Read the model definition and answer for the solid it produces. Units are mm, in the model's axes. Coordinates: 2 decimals unless noted, no trailing zeros. Answer as a JSON object with one key per item and string values. Group by question number.
1) Consider L1, parallel to Z at x = 114.3, y = -0.5; L2, parallel to Z at x = 193, y = 8. Determine where each line is inside the solid, lowest interval first.
2) Given pin 1 (9.5 mm diameter, centred on x = -38.1, z = 1047.75, fed in from -Y); pin 2 (11 mm diameter, centred on x = 38.1, z = 1047.75, fed in from -Y); pin 3 (13.5 mm diameter, centred on x = 38.1, z = 19.05, fed in from -Y), each flat-ended and moving along its own axis, determine where each tip first touches the part or whether it passes through.
3) Determine the mould class of faces 1 (the flat face through (-3, 0, 1066.8)), 2 (the flat face through (241.3, 0, 526)), 3 (the flat face through (-241.3, 0, 526)) for opening direction X: released by +X, released by -X, zero draft, split by the parting line, or undercut.
from build123d import *

# Parameters (mm, degrees)
SKETCH2_W                                         = 482.6
SKETCH2_H                                         = 38.1
BOSS_EXTRUDE1_DEPTH                               = 1066.8
CSK_FOR_5_16_FLAT_HEAD_MACHINE_SCREW1_D           = 8.4328
CSK_FOR_5_16_FLAT_HEAD_MACHINE_SCREW1_CSINK_D     = 16.129
CSK_FOR_5_16_FLAT_HEAD_MACHINE_SCREW1_CSINK_ANGLE = 82


with BuildPart() as part:
    # Sketch2 → Boss-Extrude1 (new body)
    with BuildSketch(Plane.XY):
        Rectangle(SKETCH2_W, SKETCH2_H)
    extrude(amount=BOSS_EXTRUDE1_DEPTH)

    # CSK for 5/16 Flat Head Machine Screw1 (through all)
    with Locations(Plane(origin=(0, -19.05, 0), x_dir=(-1, 0, 0), z_dir=(0, -1, 0))):
        with Locations((190.5, -1047.75), (114.3, -1047.75), (38.1, -1047.75), (-38.1, -1047.75), (-114.3, -1047.75), (-190.5, -1047.75), (114.3, -19.05), (38.1, -19.05), (-38.1, -19.05), (-114.3, -19.05), (-190.5, -19.05), (190.5, -19.05)):
            CounterSinkHole(CSK_FOR_5_16_FLAT_HEAD_MACHINE_SCREW1_D / 2, CSK_FOR_5_16_FLAT_HEAD_MACHINE_SCREW1_CSINK_D / 2, counter_sink_angle=CSK_FOR_5_16_FLAT_HEAD_MACHINE_SCREW1_CSINK_ANGLE)


solid = part.part
Worked answers:
{
 "1": {"L1": "z = 0 to 14.83, 23.27 to 1043.53, 1051.97 to 1066.8", "L2": "z = 0 to 15.65, 22.45 to 1044.35, 1051.15 to 1066.8"},
 "2": {"pin 1": "stops at y = -15.24", "pin 2": "stops at y = -16.1", "pin 3": "stops at y = -17.54"},
 "3": {"face 1": "zero draft", "face 2": "released by +X", "face 3": "released by -X"}
}
